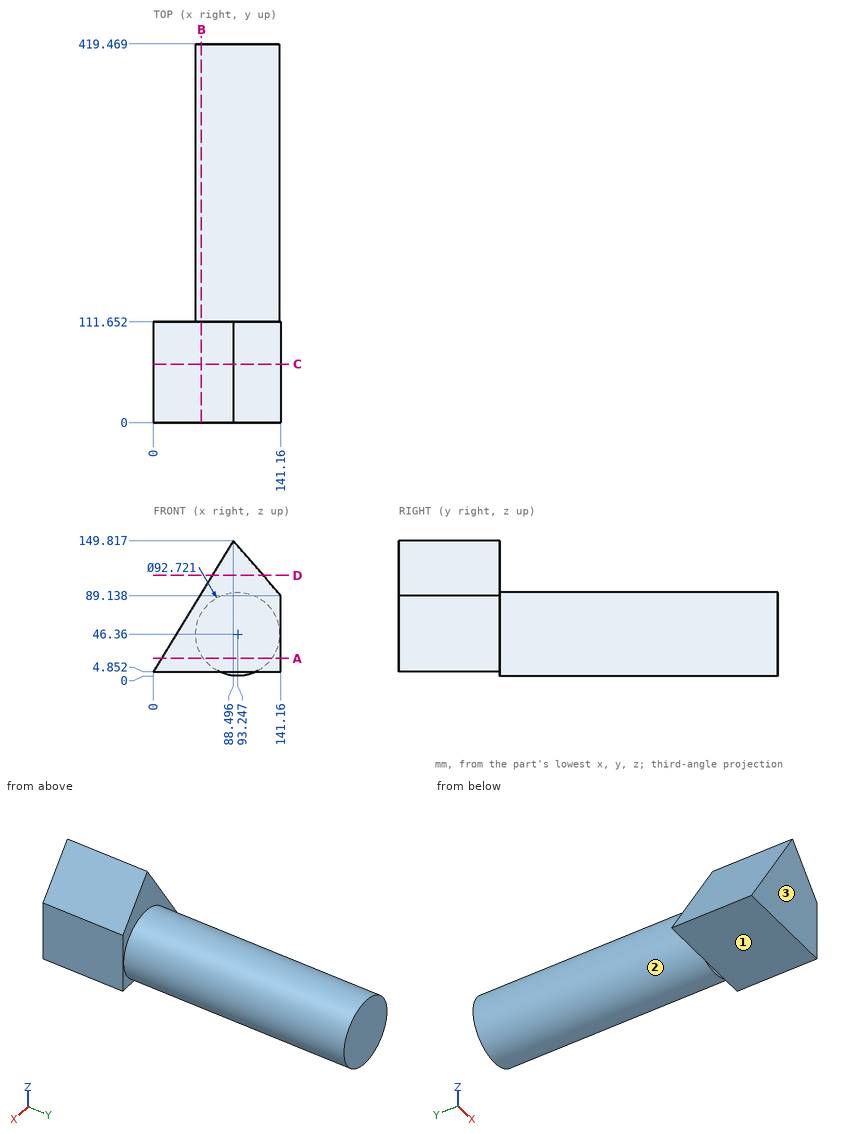
Geometry: see drawing. Coordinates: mm, zero at the bounding-box minimum. A direction names the side the tool comes from. Give positions to 0.01 mm unless a question says otherwise; leave off trailing zeros. Order: outer loops, then holes, each group sorted by start corner. A loop starts at its lowest first (then second) coordinate and runs counter-clockwise, first axis right, second up.
Q1. Section A-A on z = 19.5. Output: boundary loops of the cut face in (x, y).
Checked values:
outline: (8.94, 0) - (141.16, 0) - (141.16, 111.65) - (131.03, 111.65) - (131.03, 419.47) - (55.46, 419.47) - (55.46, 111.65) - (8.94, 111.65) - close
Q2. Section B-B on x = 53. Output: boundary loops of the cut face in (y, z), and give its area (3 significant figures).
Checked values:
outline: (0, 4.85) - (111.65, 4.85) - (111.65, 23.35) - (419.47, 23.35) - (419.47, 69.37) - (111.65, 69.37) - (111.65, 91.67) - (0, 91.67) - close
area: 23,900 mm2
Q3. Set-up query: the marked faces 1, 2 and 3. Return all of +Z, -Z, +X, -X, +Y, -Y with unobstructed straight access to the full face (end or side cutting, diameter ignored); none if empty.
Checked values:
face 1: -Z, +X, -X, -Y
face 2: +Y
face 3: +Z, -Z, +X, -X, -Y
Q4. Section D-D on z = 111.5. Output: boundary loops of the cut face in (x, y) (1 decimal).
Checked values:
outline: (65.1, 0) - (121.8, 0) - (121.8, 111.7) - (65.1, 111.7) - close
Q5. Contact query for flat-ended pins moving along their axis: pin 1 Ø5 at (x, z) = (78, 91.5) entering from -Y; pin 2 Ø12 at (y, z) = (122, 42.5) entering from +X; pin 3 Ø10 at (y, z) = (272, 93.5) entering from -X; pin 4 Ø2 at (y, z) = (266.5, 61.5) entering from +X. Output: stop coordinate, or through.
Checked values:
pin 1: stops at y = 0
pin 2: stops at x = 139.61
pin 3: stops at x = 73.92
pin 4: stops at x = 137.4
Q6. Ray query, probe 1 along Y at (x, z) = (108.5, 97.5); probe 2 along Z at (x, y) = (94, 292.5) (1 decimal); probe 3 along Z at (x, y) = (106, 270). Return the intervals inside material, ascending.
Checked values:
probe 1: y = 0 to 111.65
probe 2: z = 0 to 92.7
probe 3: z = 1.79 to 90.93
Q7. Section C-C on y = 65. Output: boundary loops of the cut face in (x, z), and give its area (3 significant figures).
Checked values:
outline: (0, 4.85) - (141.16, 4.85) - (141.16, 89.14) - (88.5, 149.82) - close
area: 12,500 mm2
